Model file for the job. Use its own axes, mm. Face numbers are marked on the shaded views. A direction names the side the tool comes from. Coordinates: 2 decimals unless noted, no trailing zeros. Write each loop counter-clockwise with the first axis right and the second up, starting at its lowest first coordinate (ties: lowest second). Pieces come first, ordered by that corner, then holes. Notation, with made-up numbers: M 70.25,71 L 129.25,71 A14 cw 129.25,80 Z; hole C -34,4 d3. An arc over 180 degrees is marked long. Put each result on its own line as item: value. Start each with the question number.
Q1. Which spindle directions (+Z, -Z, +X, -X, +Y, -Y) get a long thin tool onto all of the face, cutting with end or side? Do the marked faces 1 and 2. Say none if no direction does.
Q2. Cut at D-D (x = -12.5). Write the cut outline in (y, z).
Q3. Cut at B-B (y = 32.5). Give the number of separate pieces and of enclosed holes in the cut face, then the cut area to 3 significant figures.
Q4. Cut at A-A (z = -49.1). Write the cut outline in (x, y).
Q5. Drill centre lines: line 1 along X through (y, z) = (7.5, -37); line 2 along Z through (x, y) = (34.15, 20); line 3 along X through (y, z) = (-14.5, -72). Where is each one in solid material? Low to high.
Q6. Pull direction X, two halves, no side cores. Call the marked faces 3, 4, 5 and 6: pulls with the +X half, pulls with the -X half, needs draft (parallel to the pull), parting line crosses it, or undercut.
Q7. Cut at C-C (z = -109). Write the cut outline in (x, y).
Q8. Drop flat-ended pins along their axis: pin 1 (4.5 mm diameter, centred on x = 33, y = -37, fed in from +Z); pin 2 (10 mm diameter, centred on x = -26, y = 26, fed in from +Z); pin 3 (8 mm diameter, centred on y = -30, z = -64, fed in from -X); pin 4 (6 mm diameter, centred on x = -8, y = 23, fed in from -Z). Give the stop position or say it passes through.
Autodesk Inventor part; units mm, degrees
ref_plane "Endfläche-ProbeHeadarme" through (0, 0, -126) normal (0, 0, 1) x (1, 0, 0)
ref_plane "Z-LowerBelt" through (0, 0, -49.1) normal (0, 0, 1) x (1, 0, 0)
ref_plane "X-Belts" through (26.75, 0, 0) normal (1, 0, 0) x (0, 1, 0)
sketch "S-ProbeHead-BaseSkizze" plane through (0, 0, 0) normal (0, 0, 1) x (1, 0, 0)
  line L0 (-40, 40) -> (40, 40)
  line L1 (40, 40) -> (40, -40)
  line L2 (40, -40) -> (-40, -40)
  line L3 (-40, -40) -> (-40, 40)
  line L4 (-40, 40) -> (40, -40) construction
  line L5 (40, 40) -> (-40, -40) construction
  line L6 (-56.34, 0) -> (58.04, 0) construction
  circle A0 centre (-30, 0) radius 5
  line L7 (0, 83.0683) -> (0, -88.0384) construction
  line L8 (-7.5, 58.6245) -> (-7.5, -60.8735) construction
  line L9 (-16, 21) -> (16, 21) construction
  line L10 (16, 21) -> (16, -21) construction
  line L11 (16, -21) -> (-16, -21) construction
  line L12 (-16, -21) -> (-16, 21) construction
  line L13 (-16, 21) -> (16, -21) construction
  line L14 (16, 21) -> (-16, -21) construction
  circle A1 centre (-12.5, -10) radius 1.65
  circle A2 centre (-12.5, 10) radius 1.65
  circle A3 centre (12.5, -10) radius 1.65
  circle A4 centre (12.5, 10) radius 1.65
  line L15 (-20, 57.6709) -> (-20, -63.5946)
  line L16 (7.5, 58.6245) -> (7.5, -60.8735) construction
  line L17 (20, 57.6709) -> (20, -63.5946)
  line L18 (41.7, 25) -> (-40, 25)
  line L19 (-40, 25) -> (-40, -25)
  line L20 (-40, -25) -> (41.7, -25)
  line L21 (41.7, -25) -> (41.7, 25)
  line L22 (22, 25) -> (22, -25)
  line L23 (-22, -25) -> (-22, 25)
  point P0 (0, 0)
  point P1 (41.7, 0)
  dimension "d1" = 80
  dimension "d2" = 80
  dimension "d4" = 10
  dimension "d6" = 30
  dimension "d20" = 7.5
  dimension "d21" = 32
  dimension "d22" = 42
  dimension "d23" = 3.3
  dimension "d24" = 10
  dimension "d25" = 12.5
  dimension "d26" = 20
  dimension "d27" = 50
  dimension "d30" = 20
  dimension "d31" = 21.7
  dimension "d32" = 2
  dimension "d37" = 2
extrude "BasePlate" add sketch "S-ProbeHead-BaseSkizze" along normal blind 4 contours L18 L23 L20 L3 | L18 L17 L20 L15 | L15 L20 L23 L18 | L18 L22 L20 L17 | L18 L21 L20 L1 | L1 L20 L22 L18
ref_plane "Endfläche-ProbeHeadarme" through (0, 0, -126) normal (0, 0, 1) x (1, 0, 0)
ref_plane "ProfilDownside" through (0, 0, -56) normal (0, 0, 1) x (1, 0, 0)
extrude "Arms" add sketch "S-ProbeHead-BaseSkizze" against normal up to surface (126 mm away) contours L18 L23 L20 L3 | L18 L21 L20 L1 | L1 L20 L22 L18
ref_plane "Z-UpperBelt" through (0, 0, -36.1) normal (0, 0, 1) x (1, 0, 0)
ref_plane "Z-LowerBelt" through (0, 0, -49.1) normal (0, 0, 1) x (1, 0, 0)
ref_plane "X-Belts" through (26.75, 0, 0) normal (1, 0, 0) x (0, 1, 0)
sketch "S-Tensioners" plane through (-40, -25, 4) normal (0, -1, 0) x (1, 0, 0)
  line L0 (64.75, -47.25) -> (78.95, -47.25)
  line L1 (78.95, -47.25) -> (78.95, -58.95)
  line L2 (78.95, -58.95) -> (64.75, -58.95)
  line L3 (64.75, -58.95) -> (64.75, -47.25)
  line L4 (64.75, -47.25) -> (78.95, -58.95) construction
  line L5 (78.95, -47.25) -> (64.75, -58.95) construction
  line L6 (71.85, -74) -> (71.85, 12.5724) construction
  line L7 (-16.34, -40.1) -> (98.04, -40.1) construction
  line L8 (-16.34, -53.1) -> (98.04, -53.1) construction
  circle A0 centre (74.15, -53.1) radius 2.9
  line L9 (64.75, -34.25) -> (78.95, -34.25)
  line L10 (78.95, -34.25) -> (78.95, -45.95)
  line L11 (78.95, -45.95) -> (64.75, -45.95)
  line L12 (64.75, -45.95) -> (64.75, -34.25)
  line L13 (64.75, -34.25) -> (78.95, -45.95) construction
  line L14 (78.95, -34.25) -> (64.75, -45.95) construction
  circle A1 centre (74.15, -40.1) radius 2.9
  circle A2 centre (74.15, -40.1) radius 5
  circle A3 centre (74.15, -53.1) radius 5
  line L15 (66.75, 41.0869) -> (66.75, -158.5145) construction
  line L16 (78.95, -34.25) -> (64.75, -34.25)
  line L17 (64.75, -34.25) -> (64.75, -33.95)
  line L18 (64.75, -33.95) -> (78.95, -33.95)
  line L19 (78.95, -33.95) -> (78.95, -34.25)
  line L20 (78.95, -58.95) -> (64.75, -58.95)
  line L21 (64.75, -58.95) -> (64.75, -59.25)
  line L22 (64.75, -59.25) -> (78.95, -59.25)
  line L23 (78.95, -59.25) -> (78.95, -58.95)
  point P0 (40, -4)
  point P1 (78.95, -40.1)
  point P2 (78.95, -53.1)
  dimension "d38" = 14.2
  dimension "d39" = 11.7
  dimension "d42" = 5.8
  dimension "d43" = 14.2
  dimension "d44" = 11.7
  dimension "d45" = 5.8
  dimension "d53" = 4.8
  dimension "d54" = 4.8
  dimension "d55" = 10
  dimension "d56" = 10
  dimension "d58" = 7.4
  dimension "d59" = 7.4
  dimension "d79" = 0.3
  dimension "d80" = 0.3
extrude "Ex-Tensioners1-Holes" cut sketch "S-Tensioners" against normal blind 50 contours A0 | A1
extrude "Ex-Tensioners2-SlideVolume" cut sketch "S-Tensioners" along normal blind 35 from surface at -50 contours L0 L1 A3 L2 L3 | L2 L23 L22 L21 | L1 A3 picked at (78.3167, -53.1)
extrude "Ex-Tensioners3-SlideVolume" cut sketch "S-Tensioners" against normal blind 35 contours L17 L18 L19 L9 | L9 L10 A2 L11 L12 | L10 A2 picked at (78.3167, -40.1)
extrude "Ex-Tensioners4-SrewHead" cut sketch "S-Tensioners" against normal blind 7 contours A3 L1 | L1 A3
extrude "Ex-Tensioners5-SrewHead" cut sketch "S-Tensioners" along normal blind 7 from surface at -50 contours A2 L10 | L10 A2
sketch "S-Anschraubpunkte-ProbeAntenna" plane through (0, 0, -126) normal (0, 0, 1) x (1, 0, 0)
  line L0 (-56.34, 0) -> (58.04, 0) construction
  line L1 (0, 74.3335) -> (0, -68.3114) construction
  line L2 (41.7, 25) -> (-40, 25)
  line L3 (41.7, -25) -> (41.7, 25)
  line L4 (-40, -25) -> (41.7, -25)
  line L5 (-40, 25) -> (-40, -25)
  line L6 (41.7, 25) -> (26.7, 25)
  line L7 (26.7, 25) -> (26.7, 40)
  line L8 (26.7, 40) -> (41.7, 40)
  line L9 (41.7, 40) -> (41.7, 25)
  line L10 (22, -25) -> (22, 25)
  line L11 (22, 25) -> (22, -25)
  line L12 (-22, 25) -> (-22, -25)
  line L13 (-22, -25) -> (-22, 25)
  line L14 (41.7, 32.5) -> (26.7, 32.5) construction
  line L15 (34.2, 40) -> (34.2, 25) construction
  circle A0 centre (34.2, 32.5) radius 2.15
  circle A1 centre (34.2, 32.5) radius 4 construction
  line L16 (0.85, 53.9557) -> (0.85, -47.9335) construction
  line L17 (-40, 25) -> (-25, 25)
  line L18 (-25, 25) -> (-25, 40)
  line L19 (-25, 40) -> (-40, 40)
  line L20 (-40, 40) -> (-40, 25)
  circle A2 centre (-32.5, 32.5) radius 2.15
  circle A3 centre (-32.5, 32.5) radius 4 construction
  line L21 (41.7, -25) -> (26.7, -25)
  line L22 (26.7, -25) -> (26.7, -40)
  line L23 (26.7, -40) -> (41.7, -40)
  line L24 (41.7, -40) -> (41.7, -25)
  circle A4 centre (34.2, -32.5) radius 2.15
  circle A5 centre (34.2, -32.5) radius 4 construction
  line L25 (-40, -40) -> (-40, -25)
  line L26 (-25, -40) -> (-40, -40)
  line L27 (-40, -25) -> (-25, -25)
  line L28 (-25, -25) -> (-25, -40)
  circle A6 centre (-32.5, -32.5) radius 4 construction
  circle A7 centre (-32.5, -32.5) radius 2.15
  line L29 (34.2, 28.1987) -> (30.475, 30.3494)
  line L30 (30.475, 30.3494) -> (30.475, 40)
  line L31 (30.475, 34.6506) -> (34.2, 36.8013)
  line L32 (34.2, 36.8013) -> (37.925, 34.6506)
  line L33 (37.925, 40) -> (37.925, 30.3494)
  line L34 (37.925, 30.3494) -> (34.2, 28.1987)
  line L35 (34.2, -28.1987) -> (30.475, -30.3494)
  line L36 (30.475, -30.3494) -> (30.475, -40)
  line L37 (30.475, -34.6506) -> (34.2, -36.8013)
  line L38 (34.2, -36.8013) -> (37.925, -34.6506)
  line L39 (37.925, -40) -> (37.925, -30.3494)
  line L40 (37.925, -30.3494) -> (34.2, -28.1987)
  line L41 (-32.5, 28.1987) -> (-28.775, 30.3494)
  line L42 (-28.775, 30.3494) -> (-28.775, 40)
  line L43 (-28.775, 34.6506) -> (-32.5, 36.8013)
  line L44 (-32.5, 36.8013) -> (-36.225, 34.6506)
  line L45 (-36.225, 40) -> (-36.225, 30.3494)
  line L46 (-36.225, 30.3494) -> (-32.5, 28.1987)
  line L47 (-36.225, -40) -> (-36.225, -30.3494)
  line L48 (-32.5, -36.8013) -> (-36.225, -34.6506)
  line L49 (-28.775, -34.6506) -> (-32.5, -36.8013)
  line L50 (-28.775, -30.3494) -> (-28.775, -40)
  line L51 (-32.5, -28.1987) -> (-28.775, -30.3494)
  line L52 (-36.225, -30.3494) -> (-32.5, -28.1987)
  point P0 (0, 0)
  dimension "d46" = 50
  dimension "d67" = 15
  dimension "d68" = 15
  dimension "d69" = 4.3
  dimension "d70" = 8
  dimension "d71" = 81.7
  dimension "d72" = 40.85
  dimension "d75" = 65
  dimension "d76" = 66.7
  dimension "d81" = 7.45
extrude "Ex-Anschraubpunkte-Eb1" add sketch "S-Anschraubpunkte-ProbeAntenna" along normal blind 2 contours L2 L7 L8 L30 L29 L34 L33 L9 | L24 L23 L39 L40 L35 L36 L22 L4 | L33 L32 L31 L30 L8 | L23 L36 L37 L38 L39 | L33 L34 L29 L30 L31 L32 | L2 L20 L19 L45 L46 L41 L42 L18 | L38 L37 L36 L35 L40 L39 | L28 L26 L50 L51 L52 L47 L25 L4 | L42 L43 L44 L45 L19 | L42 L41 L46 L45 L44 L43 | L26 L47 L48 L49 L50 | L49 L48 L47 L52 L51 L50
extrude "Ex-Anschraubpunkte-Eb2" add sketch "S-Anschraubpunkte-ProbeAntenna" along normal blind 2 from surface at 2 contours L2 L7 L8 L30 L29 L34 L33 L9 | L24 L23 L39 L40 L35 L36 L22 L4 | L33 L32 L31 L30 L8 | L23 L36 L37 L38 L39 | L2 L20 L19 L45 L46 L41 L42 L18 | L28 L26 L50 L51 L52 L47 L25 L4 | L42 L43 L44 L45 L19 | L26 L47 L48 L49 L50
extrude "Ex-Anschraubpunkte-Eb3" add sketch "S-Anschraubpunkte-ProbeAntenna" along normal blind 3.1 from surface at 4 contours L2 L7 L8 L30 L29 L34 L33 L9 | L24 L23 L39 L40 L35 L36 L22 L4 | L2 L20 L19 L45 L46 L41 L42 L18 | L28 L26 L50 L51 L52 L47 L25 L4
extrude "Ex-Anschraubpunkte-Eb4" add sketch "S-Anschraubpunkte-ProbeAntenna" along normal blind 1 from surface at 7.1 contours L2 L7 L8 L30 L29 L34 L33 L9 | L24 L23 L39 L40 L35 L36 L22 L4 | L33 L32 L31 L30 L8 | L23 L36 L37 L38 L39 | L33 L34 L29 L30 L31 L32 | L2 L20 L19 L45 L46 L41 L42 L18 | L38 L37 L36 L35 L40 L39 | L28 L26 L50 L51 L52 L47 L25 L4 | L42 L43 L44 L45 L19 | L42 L41 L46 L45 L44 L43 | L26 L47 L48 L49 L50 | L49 L48 L47 L52 L51 L50
ref_plane "Anschraubpunkt-Spiegelebene" through (0.85, 53.9557, -126) normal (-1, 0, 0) x (0, -1, 0)
ref_plane "ProfilTopSide" through (0, 0, -16) normal (0, 0, 1) x (1, 0, 0)
equation "\"d43\" = d38"
equation "\"d44\" = d39"
equation "\"d45\" = d42"
equation "\"d53\" = d54"
equation "\"d55\" = d56"
equation "\"d58\" = d59"
equation "\"d80\" = d79"
equation "\"d72\" = 0.5 * d71"
properties part number "ProbeHead-BaseBody V2"
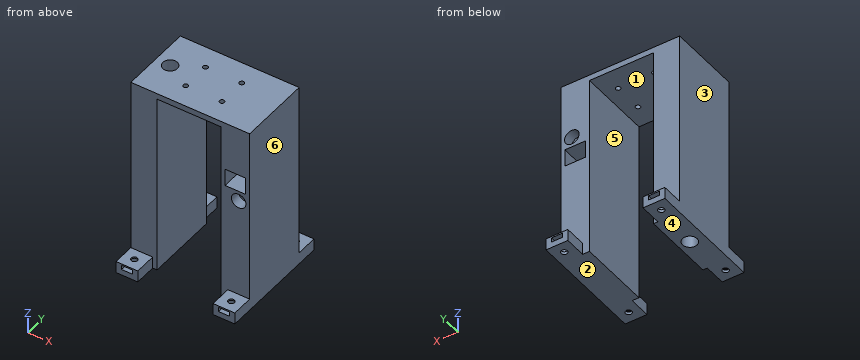
Computed values:
1. face 1: -Z, +Y, -Y
1. face 2: -Z, +X, -X, +Y, -Y
2. outline: M -25,0 L -11.65,0 L -11.65,4 L -25,4 Z; M -8.35,0 L 8.35,0 L 8.35,4 L -8.35,4 Z; M 11.65,0 L 25,0 L 25,4 L 11.65,4 Z
3. separate pieces: 4
3. enclosed holes: 0
3. area: 141 mm2
4. outline: M -40,-25 L -22,-25 L -22,25 L -40,25 Z; M 22,-25 L 29.15,-25 L 29.15,-18 L 31.25,-18 L 31.25,-10 L 24.75,-10 L 24.75,25 L 22,25 Z; M 37.05,-18 L 39.15,-18 L 39.15,-25 L 41.7,-25 L 41.7,25 L 38.95,25 L 38.95,-10 L 37.05,-10 Z; hole C -30,0 d10
5. line 1: -40 to -22, 22 to 24.75, 38.95 to 41.7
5. line 2: -126 to -55.25, -43.25 to -41.1, -31.1 to 4
5. line 3: -40 to -22, 22 to 41.7
6. face 3: pulls with the -X half
6. face 4: needs draft
6. face 5: undercut
6. face 6: pulls with the +X half
7. outline: M -40,-25 L -22,-25 L -22,25 L -40,25 Z; M 22,-25 L 41.7,-25 L 41.7,25 L 22,25 Z; hole C -30,0 d10
8. pin 1: z = -117.9
8. pin 2: z = 4
8. pin 3: through
8. pin 4: z = 0
